Source: CAD feature listing. Evaluate the final solid. Frame: model axes, mm. Face numbers are marked on the shaded views. Round coordinates to 2 decimals unless told otherwise and drop trailing zeros. Use a Markdown table: item, result.
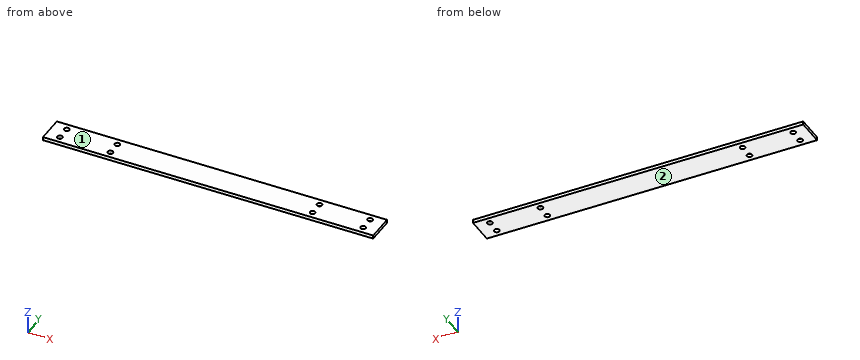
Autodesk Inventor part; units mm, degrees
ref_plane "YZ Plane" through (0, 0, 0) normal (1, 0, 0) x (0, 1, 0)
ref_plane "XZ Plane" through (0, 0, 0) normal (0, 1, 0) x (-1, 0, 0)
ref_plane "XY Plane" through (0, 0, 0) normal (0, 0, 1) x (1, 0, 0)
sketch "Sketch1" plane through (0, 0, 0) normal (0, 0, 1) x (1, 0, 0)
  line L0 (155.575, 12.7) -> (-155.575, 12.7)
  line L1 (-155.575, 12.7) -> (-155.575, -12.7)
  line L2 (-155.575, -12.7) -> (155.575, -12.7)
  line L3 (155.575, -12.7) -> (155.575, 12.7)
  line L4 (155.575, 12.7) -> (-155.575, -12.7) construction
  line L5 (-155.575, 12.7) -> (155.575, -12.7) construction
  line L6 (-149.225, 12.7) -> (-136.525, 12.7)
  line L7 (-136.525, 12.7) -> (-136.525, -12.7)
  line L8 (-136.525, -12.7) -> (-149.225, -12.7)
  line L9 (-149.225, -12.7) -> (-149.225, 12.7)
  circle A0 centre (-142.875, 6.35) radius 2.4257
  circle A1 centre (-142.875, -6.35) radius 2.4257
  line L10 (149.225, 12.7) -> (136.525, 12.7)
  line L11 (136.525, 12.7) -> (136.525, -12.7)
  line L12 (136.525, -12.7) -> (149.225, -12.7)
  line L13 (149.225, -12.7) -> (149.225, 12.7)
  circle A2 centre (142.875, 6.35) radius 2.4257
  circle A3 centre (142.875, -6.35) radius 2.4257
  line L14 (101.6, 12.7) -> (88.9, 12.7)
  line L15 (88.9, 12.7) -> (88.9, -12.7)
  line L16 (88.9, -12.7) -> (101.6, -12.7)
  line L17 (101.6, -12.7) -> (101.6, 12.7)
  line L18 (-101.6, 12.7) -> (-88.9, 12.7)
  line L19 (-88.9, 12.7) -> (-88.9, -12.7)
  line L20 (-88.9, -12.7) -> (-101.6, -12.7)
  line L21 (-101.6, -12.7) -> (-101.6, 12.7)
  circle A4 centre (-95.25, 6.35) radius 2.4257
  circle A5 centre (-95.25, -6.35) radius 2.4257
  circle A6 centre (95.25, -6.35) radius 2.4257
  circle A7 centre (95.25, 6.35) radius 2.4257
  point P0 (0, 0)
  point P1 (149.225, 0)
  dimension "d0" = 311.15
  dimension "d1" = 25.4
  dimension "d2" = 12.7
  dimension "d3" = 6.35
  dimension "d4" = 4.8514
  dimension "d5" = 4.8514
  dimension "d6" = 6.35
  dimension "d7" = 6.35
  dimension "d8" = 12.7
  dimension "d9" = 6.35
  dimension "d10" = 4.8514
  dimension "d11" = 4.8514
  dimension "d12" = 12.7
  dimension "d13" = 47.625
  dimension "d14" = 12.7
  dimension "d15" = 47.625
  dimension "d16" = 4.8514
  dimension "d17" = 4.8514
  dimension "d18" = 4.8514
  dimension "d19" = 4.8514
  dimension "d22" = 6.35
  dimension "d23" = 6.35
  dimension "d24" = 6.35
  dimension "d25" = 6.35
  dimension "d26" = 6.35
  dimension "d27" = 6.35
  dimension "d28" = 6.35
  dimension "d29" = 6.35
extrude "Extrusion1" add sketch "Sketch1" along normal blind 3.175
properties part number "Chassis Bar" material "Stainless Steel"
Q1. Section A-A on z = 1.75. Give the number of separate pieces and of enclosed holes in the cut face, plus the area to 3 significant figures.
Results are:
| item | result |
|---|---|
| separate pieces | 1 |
| enclosed holes | 8 |
| area | 7,760 mm^2 |
Q2. Mould query, pull axis Z, two halves, no side actions, for the marked faces 1 and 2. Classes: +Z half, -Z half, draft (parallel to the pull), parting line (faces both ways), or undercut.
Results are:
| item | result |
|---|---|
| face 1 | +Z half |
| face 2 | -Z half |
Q3. First-contact query: pin 1 Ø3 at (x, y) = (-95.25, -6.35) entering from -Z. Flat tip, straight axial feed; report the tip coordinate or a pass-through.
Results are:
| item | result |
|---|---|
| pin 1 | through |
Q4. Line query: L1, parallel to Y at x = 95.25, z = 0.7; L2, parallel to X at y = 5.5, z = 2.2 (3 decimals); L3, parallel to X at y = -4.5, z = 1.4 (3 decimals). Output: solid intervals per line, ascending.
Results are:
| item | result |
|---|---|
| L1 | -12.7 to -8.78, -3.92 to 3.92, 8.78 to 12.7 |
| L2 | -155.575 to -145.147, -140.603 to -97.522, -92.978 to 92.978, 97.522 to 140.603, 145.147 to 155.575 |
| L3 | -155.575 to -144.444, -141.306 to -96.819, -93.681 to 93.681, 96.819 to 141.306, 144.444 to 155.575 |
